```python
from build123d import *

# Parameters (mm, degrees)
SKETCH1_W           = 20.32
SKETCH1_H           = 20.32
BOSS_EXTRUDE1_DEPTH = 3
SKETCH2_W           = 13.085786438
SKETCH2_H           = 15.522266203
BOSS_EXTRUDE2_DEPTH = 3
SKETCH5_W           = 31.587668609
SKETCH5_H           = 25.562972936
CUT_EXTRUDE1_DEPTH  = 0.1
SKETCH6_W           = 20.32
SKETCH6_H           = 3.606
CUT_EXTRUDE2_DEPTH  = 10
SKETCH7_R           = 1.6
CUT_EXTRUDE3_DEPTH  = 10
SKETCH8_R           = 1.6
CUT_EXTRUDE4_DEPTH  = 10


with BuildPart() as part:
    # Sketch1 → Boss-Extrude1 (new body)
    with BuildSketch(Plane(origin=(0, 0, 0), x_dir=(1, 0, 0), z_dir=(0, 1, 0))):
        with Locations((10.16, 10.16)):
            Rectangle(SKETCH1_W, SKETCH1_H)
    extrude(amount=BOSS_EXTRUDE1_DEPTH)

    # Sketch2 → Boss-Extrude2 (add)
    with BuildSketch(Plane(origin=(20.32, 0, 0), x_dir=(0, 0, -1), z_dir=(1, 0, 0))):
        with Locations((10.171106781, -4.720966496)):
            Rectangle(SKETCH2_W, SKETCH2_H)
    extrude(amount=-BOSS_EXTRUDE2_DEPTH)

    # Sketch5 → Cut-Extrude1 (cut)
    with BuildSketch(Plane(origin=(0, 3.040166606, 0), x_dir=(1, 0, 0), z_dir=(0, 1, 0))):
        with Locations((13.28189867, 9.26803237)):
            Rectangle(SKETCH5_W, SKETCH5_H)
    extrude(amount=-CUT_EXTRUDE1_DEPTH, mode=Mode.SUBTRACT)

    # Sketch6 → Cut-Extrude2 (cut)
    with BuildSketch(Plane(origin=(0, 0, 0), x_dir=(-1, 0, 0), z_dir=(0, -1, 0))):
        with Locations((-10.16, 18.517)):
            Rectangle(SKETCH6_W, SKETCH6_H)
    extrude(amount=-CUT_EXTRUDE2_DEPTH, mode=Mode.SUBTRACT)

    # Sketch7 → Cut-Extrude3 (cut)
    with BuildSketch(Plane(origin=(0, 2.940166606, 0), x_dir=(1, 0, 0), z_dir=(0, 1, 0))):
        with Locations(Location((5.37, 4.15, 0), (0, 0, 270))):
            Circle(SKETCH7_R)
        with Locations(Location((15.27, 4.15, 0), (0, 0, 270))):
            Circle(SKETCH7_R)
    extrude(amount=-CUT_EXTRUDE3_DEPTH, mode=Mode.SUBTRACT)

    # Sketch8 → Cut-Extrude4 (cut)
    with BuildSketch(Plane.ZY.offset(-17.32)):
        with Locations((-10.232213562, -9.006524303)):
            Circle(SKETCH8_R)
        with Locations((-10.228213562, -3.127074003)):
            Circle(SKETCH8_R)
    extrude(amount=-CUT_EXTRUDE4_DEPTH, mode=Mode.SUBTRACT)


solid = part.part
```
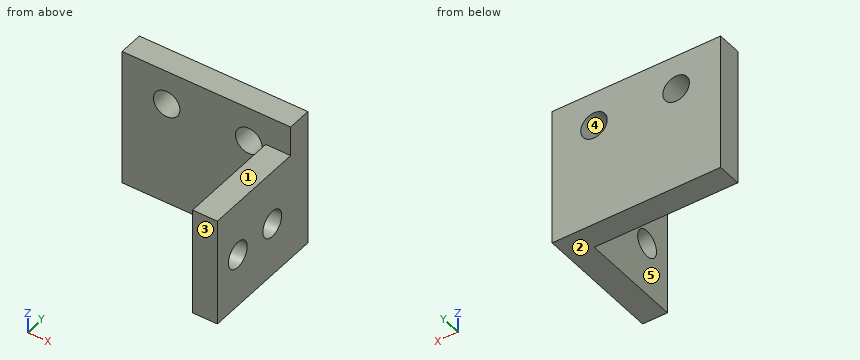
Geometry check sheet. Reference: the model listing, model coordinates, mm. Face numbers are marked on the shaded views. A direction names the side the tool comes from. Give positions to 0.01 mm unless a question says otherwise; leave off trailing zeros. Loops run counter-clockwise (first coordinate to the right, second up) from the corner with the lowest first, then second, coordinate; pieces in that order, holes last. Notation, with made-up numbers: M 61,36.25 L 71,36.25 A16 ccw 71,66.25 Z; hole C -1,35.25 d3. An arc over 180 degrees is marked long. Answer as CSV lines item,"result".
Item 1: Cross-section at D-D on z = -13. Record the cut outline in (x, y), and give its area (3 significant figures).
Values:
outline,"M 0,0 L 17.32,0 L 17.32,-12.48 L 20.32,-12.48 L 20.32,2.94 L 0,2.94 Z"
area,"97.2 mm²"
Item 2: Cross-section at A-A on z = -4.15. Record the cut outline in (x, y), and give its area (3 significant figures).
Values:
outline,"M 0,0 L 3.77,0 L 3.77,2.94 L 0,2.94 Z; M 6.97,0 L 13.67,0 L 13.67,2.94 L 6.97,2.94 Z; M 16.87,0 L 17.32,0 L 17.32,-12.48 L 20.32,-12.48 L 20.32,2.94 L 16.87,2.94 Z"
area,"78.4 mm²"
Item 3: Material ranges on line 1 (X direction, y = 2.1, z = -4.15); line 2 (Y direction, x = 12.25, z = -15.25); line 3 (X direction, y = -1.25, z = -10.25), recorded low to high.
Values:
line 1,"x = 0 to 3.77, 6.97 to 13.67, 16.87 to 20.32"
line 2,"y = 0 to 2.94"
line 3,"x = 17.32 to 20.32"
Item 4: Cross-section at C-C on y = -2.5. Record the cut outline in (x, z), and give its area (3 significant figures).
Values:
outline,"M 17.32,-16.71 L 20.32,-16.71 L 20.32,-11.7 L 17.32,-11.7 Z; M 17.32,-8.76 L 20.32,-8.76 L 20.32,-3.63 L 17.32,-3.63 Z"
area,"30.4 mm²"
Item 5: Depth check by flat-ended pin: P1, Ø3.5, axis at x = 19, y = -5, coming from the +Z side; P2, Ø4, axis at x = 15.27, z = -4.15, coming from the -Y side; P3, Ø1, axis at y = -3, z = -12, coming from the -X side. Enter the tip coordinate at first touch or a pass-through.
Values:
P1,"stops at z = -3.63"
P2,"stops at y = 0"
P3,"stops at x = 17.32"
Item 6: Access from +Z, -Z, +X, -X, +Y, -Y to the whole of each face (thin tool, end or side, straight path). Record for the marked faces 1 and 2.
Values:
face 1,"+Z, +X, -X, -Y"
face 2,"-Z, +X, -X, +Y, -Y"
Item 7: Cross-section at B-B on x = 5.37. Record the cut outline in (y, z), and give its area (3 significant figures).
Values:
outline,"M 0,-16.71 L 2.94,-16.71 L 2.94,-5.75 L 0,-5.75 Z; M 0,-2.55 L 2.94,-2.55 L 2.94,0 L 0,0 Z"
area,"39.7 mm²"
Item 8: Release check for a two-part mould opening along X. For the marked faces 3, 4 and 5 record: pulls with the +X half, pulls with the -X half, needs draft (parallel to the pull), parting line crosses it, or undercut.
Values:
face 3,"needs draft"
face 4,"undercut"
face 5,"pulls with the -X half"
